```python
from build123d import *

# Parameters (mm, degrees)
BOSS_EXTRUDE1_DEPTH = 60
FILLET1_R           = 10
SKETCH2_R           = 5
CUT_EXTRUDE1_DEPTH  = 60


with BuildPart() as part:
    # Sketch1 → Boss-Extrude1 (new body)
    with BuildSketch(Plane.XY):
        Polygon((-86.358974359, -10), (-83.530547234, -12.828427125), (-43.530547234, 27.171572875), (-6.358974359, 27.171572875), (-6.358974359, 31.171572875), (-45.187401484, 31.171572875), align=None)
    extrude(amount=BOSS_EXTRUDE1_DEPTH)

    # Fillet1
    fillet1_edges = [part.edges().sort_by_distance(p)[0] for p in [
        (-45.187401484, 31.171572875, 30),
        (-43.530547234, 27.171572875, 30),
    ]]
    fillet(fillet1_edges, radius=FILLET1_R)

    # Sketch2 → Cut-Extrude1 (cut)
    with BuildSketch(Plane(origin=(0, 31.171572875, 0), x_dir=(1, 0, 0), z_dir=(0, 1, 0))):
        with Locations(Location((-21.358974359, -30, 0), (0, 0, 180))):
            Circle(SKETCH2_R)
    extrude(amount=-CUT_EXTRUDE1_DEPTH, mode=Mode.SUBTRACT)


solid = part.part
```
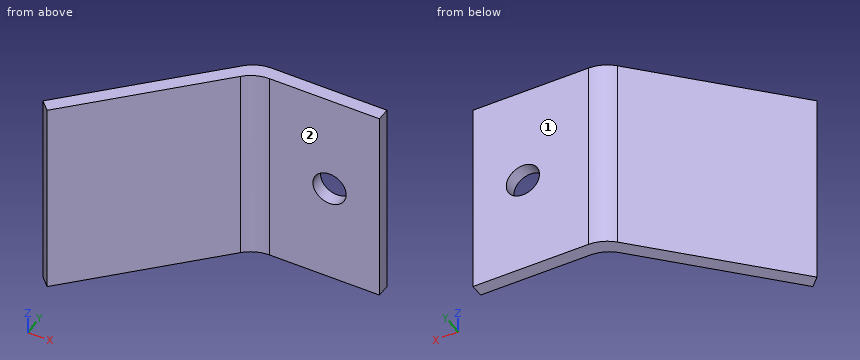
Check sheet for the modelled part. Datum: model origin and axes. Units: mm. Face numbers are marked on the shaded views. A direction names the side the tool comes from. Round coordinates to 2 decimals unless told otherwise and drop trailing zeros. Loops run counter-clockwise (first coordinate to the right, second up) from the corner with the lowest first, then second, coordinate; pieces in that order, holes last. Notation, with made-up numbers: (-27, 63) -> (9, 63) arc R17 cw to (9, 68) -> close; hole circle Ø9 at (76.25, 46.25). An arc over 180 degrees is marked (long way). Answer in a Markdown table with one row per item.
Q1. Sectioned sample at C-C on x = -30. Enter the section's corners in (y, z), then the cut area to 3 significant figures.
Data:
| item | result |
|---|---|
| outline | (27.17, 0) -> (31.17, 0) -> (31.17, 60) -> (27.17, 60) -> close |
| area | 240 mm^2 |
Q2. Go/stop test with flat-tipped pins: P1, Ø5, axis at x = -53.5, z = 22, coming from the -Y side; P2, Ø16.5, axis at x = -23.5, z = 41.5, coming from the -Y side; P3, Ø10, axis at x = -74, z = 18.5, coming from the +Y side. Record where each tip stops, or that it passes through.
Data:
| item | result |
|---|---|
| P1 | stops at y = 14.7 |
| P2 | stops at y = 27.17 |
| P3 | stops at y = 7.36 |
Q3. Sectioned sample at A-A on z = 30. Enter the section's corners in (x, y), then the cut area to 3 significant figures.
Data:
| item | result |
|---|---|
| outline | (-86.36, -10) -> (-83.53, -12.83) -> (-46.46, 24.24) arc R10 cw to (-39.39, 27.17) -> (-26.36, 27.17) -> (-26.36, 31.17) -> (-41.05, 31.17) arc R10 ccw to (-48.12, 28.24) -> close; (-16.36, 27.17) -> (-6.36, 27.17) -> (-6.36, 31.17) -> (-16.36, 31.17) -> close |
| area | 342 mm^2 |
Q4. Sectioned sample at B-B on z = 11. Enter the section's corners in (x, y), then the cut area to 3 significant figures.
Data:
| item | result |
|---|---|
| outline | (-86.36, -10) -> (-83.53, -12.83) -> (-46.46, 24.24) arc R10 cw to (-39.39, 27.17) -> (-6.36, 27.17) -> (-6.36, 31.17) -> (-41.05, 31.17) arc R10 ccw to (-48.12, 28.24) -> close |
| area | 382 mm^2 |
Q5. Set-up check for the marked faces 1 and 2: record each of +Z, -Z, +X, -X, +Y, -Y from which the full face is reachable in a straight line by a thin tool's end or side.
Data:
| item | result |
|---|---|
| face 1 | +Z, -Z, +X, -X, +Y |
| face 2 | +Z, -Z, +X, -Y |
Q6. Sectioned sample at D-D on y = 26. Enter the section's corners in (x, z), then the cut area to 3 significant figures.
Data:
| item | result |
|---|---|
| outline | (-50.36, 0) -> (-44.09, 0) -> (-44.09, 60) -> (-50.36, 60) -> close |
| area | 376 mm^2 |
Q7. Thickness scan on L1, parallel to Y at x = -36.5, z = 34; L2, parallel to X at y = -8, z = 28.5; L3, parallel to Y at x = -41.5, z = 47.5. Record the ranges inside material, lowest first.
Data:
| item | result |
|---|---|
| L1 | y = 27.17 to 31.17 |
| L2 | x = -84.36 to -78.7 |
| L3 | y = 26.95 to 31.16 |
